Study the drawing (mm; zero at the part's minimum x, y, z) and answer. A direction names the side the tool comes from. Round coordinates to 2 decimals unless told otherwise and drop trailing zeros. Order: outer loops, then holes, each group sorted by start corner. A loop starts at its lowest first (then second) coordinate and runs counter-clockwise, first axis right, second up. Notation, with made-up numbers: (-24.5, -10.75) - (0.5, -10.75) arc R15 cw to (0.5, 4.25) - close; hole circle Ø4 at (-7.75, 26). An arc over 180 degrees is marked (long way). Put each result on its own line as item: value. Start each with the question number.
Q1. Section A-A on y = 2.25 is taken. Give the vertices of the cut face in (x, z).
Q2. Find the intervals of material crossed by line 1 along Z through (x, y) = (13.5, 1.75); line 2 along X through (y, z) = (14, 22); line 3 along Y through (x, z) = (14.5, 34), in increasing order. Write a range as from..to.
Q3. Which of the six approach directions +Z, -Z, +X, -X, +Y, -Y give full straight-line access (tool end or side, diameter ignored) to the marked faces 5, 6 and 7?
Q4. For a pull along Z with two mould halves and no side action, classify the marked faces 1, 2, 3 and 4 as pulls with the +Z half, pulls with the -Z half, needs draft (parallel to the pull), parting line crosses it, or undercut.
Q5. Section C-C on x = 16.5 is taken. Give the vertices of the cut face in (y, z), then the cut area to 3 significant figures.
Q6. Each of these flat-tipped pins is pushed along its axis until it touches: pin 1 Ø4 at (x, y) = (12, 16) entering from +Z; pin 2 Ø10 at (x, z) = (3.5, 13.5) entering from +Y; pin 3 Ø2.5 at (x, z) = (5.5, 5.5) entering from -Y. Where does it stop, or does it pass through?
Q7. Section D-D on x = 10.25 is taken. State how many separate pieces and enclosed holes the cut face has, then the cut area to 3 significant figures.
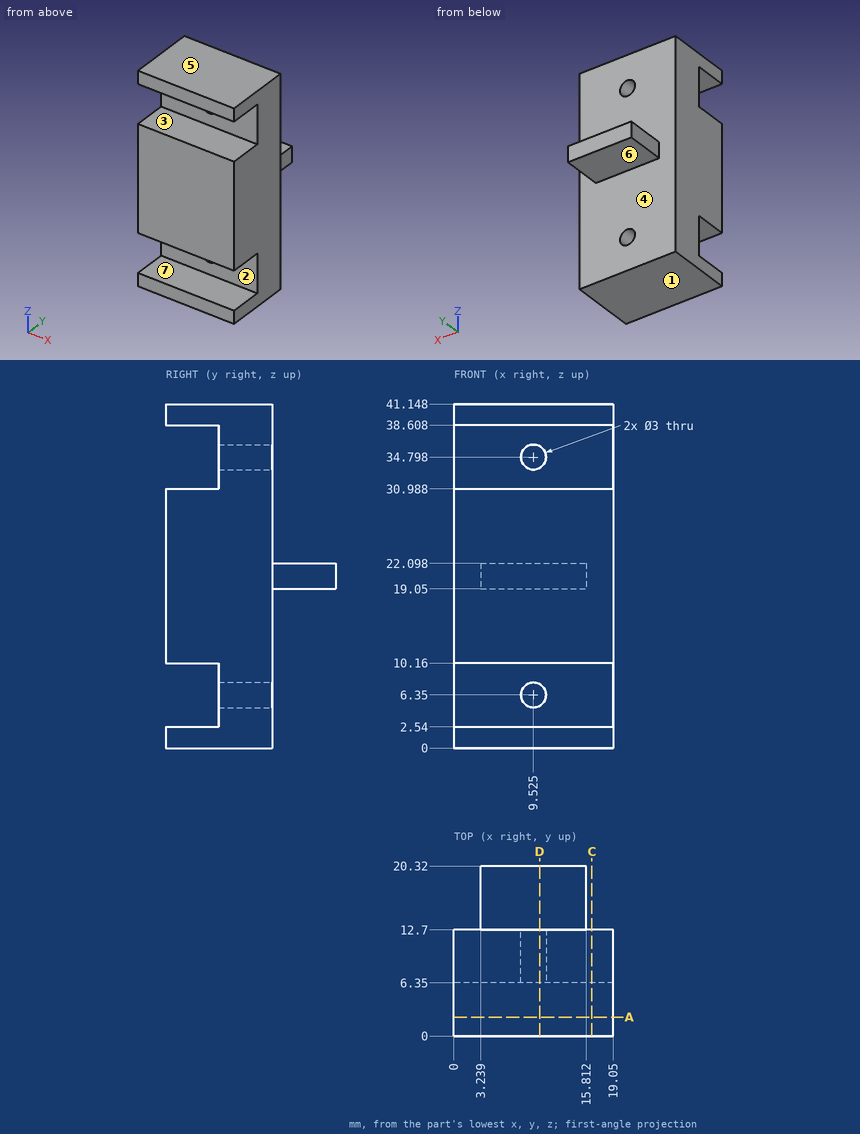
Findings:
1. outline: (0, 0) - (19.05, 0) - (19.05, 2.54) - (0, 2.54) - close; (0, 10.16) - (19.05, 10.16) - (19.05, 30.99) - (0, 30.99) - close; (0, 38.61) - (19.05, 38.61) - (19.05, 41.15) - (0, 41.15) - close
2. line 1: 0..2.54, 10.16..30.99, 38.61..41.15
2. line 2: 3.24..15.81
2. line 3: 6.35..12.7
3. face 5: +Z, +X, -X, +Y, -Y
3. face 6: -Z, +X, -X, +Y
3. face 7: +X, -X, -Y
4. face 1: pulls with the -Z half
4. face 2: undercut
4. face 3: undercut
4. face 4: needs draft
5. outline: (0, 0) - (12.7, 0) - (12.7, 41.15) - (0, 41.15) - (0, 38.61) - (6.35, 38.61) - (6.35, 30.99) - (0, 30.99) - (0, 10.16) - (6.35, 10.16) - (6.35, 2.54) - (0, 2.54) - close
5. area: 426 mm2
6. pin 1: z = 22.1
6. pin 2: y = 12.7
6. pin 3: y = 6.35
7. separate pieces: 3
7. enclosed holes: 0
7. area: 416 mm2
